Source: CAD feature listing. Evaluate the final solid. Frame: model axes, mm. Face numbers are marked on the shaded views. A direction names the side the tool comes from. Give positions to 0.01 mm unless a question says otherwise; leave off trailing zeros. Order: outer loops, then holes, each group sorted by start corner. A loop starts at its lowest first (then second) coordinate and runs counter-clockwise, first axis right, second up.
from build123d import *

# Parameters (mm, degrees)
SWEEP1_PROFILE_R = 0.8


with BuildPart() as part:
    # Sweep1: sweep along a path in Sketch1
    with BuildLine(Plane(origin=(0, 0, 0), x_dir=(1, 0, 0), z_dir=(0, 1, 0))) as sweep1_path:
        Line((11.95, 0), (11.95, -10.4))
        ThreePointArc((11.95, -10.4), (11.657106781, -11.107106781), (10.95, -11.4))
        Line((10.95, -11.4), (-10.95, -11.4))
        ThreePointArc((-10.95, -11.4), (-11.657106781, -11.107106781), (-11.95, -10.4))
        Line((-11.95, -10.4), (-11.95, 0))
    # Sweep1 profile (on start of the path) → Sweep1 (sweep)
    with BuildSketch(Plane(origin=(11.95, 0, 0), x_dir=(1, 0, 0), z_dir=(0, 0, 1))):
        Circle(SWEEP1_PROFILE_R)
    sweep(path=sweep1_path.line)


solid = part.part
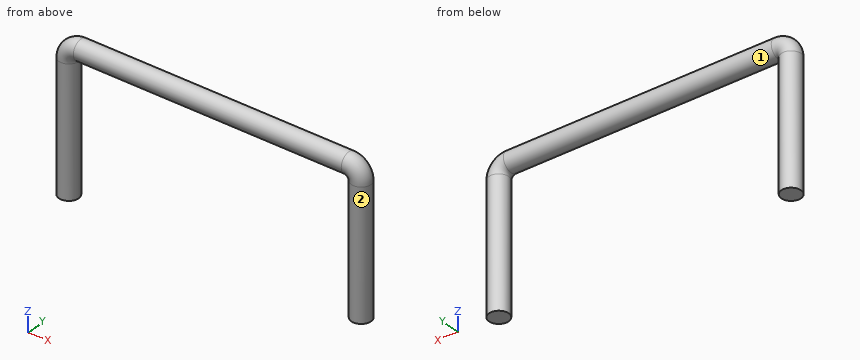
1) Section query C-C on x = 8.25. Output: boundary loops of the cut face in (y, z).
Checks:
outline: circle Ø1.6 at (0, 11.4)
2) Section query B-B on z = 2.5. Output: boundary loops of the cut face in (x, y), and give its area (3 significant figures).
Checks:
outline: circle Ø1.6 at (-11.95, 0); circle Ø1.6 at (11.95, 0)
area: 4.02 mm2
3) Section query A-A on y = 0. Output: boundary loops of the cut face in (x, z), and give its area (3 significant figures).
Checks:
outline: (-12.75, 0) - (-11.15, 0) - (-11.15, 10.4) arc R0.2 cw to (-10.95, 10.6) - (10.95, 10.6) arc R0.2 cw to (11.15, 10.4) - (11.15, 0) - (12.75, 0) - (12.75, 10.4) arc R1.8 ccw to (10.95, 12.2) - (-10.95, 12.2) arc R1.8 ccw to (-12.75, 10.4) - close
area: 73.3 mm2
4) Reachability of the marked faces 1 and 2 from +Z, -Z, +X, -X, +Y, -Y: full face, straight path, thin tool, end or side. Return the list, or none.
Checks:
face 1: none
face 2: -Z
5) Ray query, L1, parallel to X at y = 0.1, z = 8.25; L2, parallel to X at y = 0.7, z = 5.75; L3, parallel to Z at x = 5.75, y = 0. Return the intervals inside material, ascending.
Checks:
L1: x = -12.74 to -11.16, 11.16 to 12.74
L2: x = -12.34 to -11.56, 11.56 to 12.34
L3: z = 10.6 to 12.2
